from build123d import *

# Parameters (mm, degrees)
SALIENTE_EXTRUIR1_DEPTH    = 10
REDONDEO1_R                = 0.5
REDONDEO2_R                = 0.5
CROQUIS3_W                 = 6.24
CROQUIS3_H                 = 1.8
SALIENTE_EXTRUIR2_DEPTH    = 10
CROQUIS2_R                 = 1.5
CORTAR_EXTRUIR1_DEPTH      = 2.8
CORTAR_EXTRUIR1_DEPTH_BACK = 5.3


with BuildPart() as part:
    # Croquis1 → Saliente-Extruir1 (new body)
    with BuildSketch(Plane(origin=(0, 0, 0), x_dir=(-1, 0, 0), z_dir=(0, 0, 1))):
        Polygon((4.5, -1.799339828), (4.5, -3.439339828), (7.16, -6.099339828), (9.75, -6.099339828), (12.84, -6.099339828), (15.5, -3.439339828), (15.5, -1.799339828), align=None)
    extrude(amount=SALIENTE_EXTRUIR1_DEPTH)

    # Redondeo1
    redondeo1_edges = [part.edges().sort_by_distance(p)[0] for p in [
        (-15.5, 1.799339828, 5),
    ]]
    fillet(redondeo1_edges, radius=REDONDEO1_R)

    # Redondeo2
    redondeo2_edges = [part.edges().sort_by_distance(p)[0] for p in [
        (-15.5, 3.439339828, 5),
        (-12.84, 6.099339828, 5),
        (-7.16, 6.099339828, 5),
        (-4.5, 3.439339828, 5),
        (-4.5, 1.799339828, 5),
    ]]
    fillet(redondeo2_edges, radius=REDONDEO2_R)

    # Croquis3 → Saliente-Extruir2 (add)
    with BuildSketch(Plane.XY.offset(10)):
        with Locations((-10, 0.899339828)):
            Rectangle(CROQUIS3_W, CROQUIS3_H)
    extrude(amount=-SALIENTE_EXTRUIR2_DEPTH)

    # Croquis2 → Cortar-Extruir1 (cut, two sides)
    with BuildSketch(Plane(origin=(0, 1.799339828, 0), x_dir=(-1, 0, 0), z_dir=(0, -1, 0))) as cortar_extruir1_sk:
        with Locations((10, -5)):
            Circle(CROQUIS2_R)
    extrude(amount=CORTAR_EXTRUIR1_DEPTH, mode=Mode.SUBTRACT)
    extrude(cortar_extruir1_sk.sketch, amount=-CORTAR_EXTRUIR1_DEPTH_BACK, mode=Mode.SUBTRACT)


solid = part.part
Read the model definition and answer for the solid it produces. Units are mm, in the model's axes. A direction names the side the tool comes from. Give positions to 0.01 mm unless a question says otherwise; leave off trailing zeros. Write each loop counter-clockwise with the first axis right and the second up, starting at its lowest first coordinate (ties: lowest second). Pieces come first, ordered by that corner, then holes. Notation, with made-up numbers: M 61,71 L 108,71 A31 ccw 108,101 Z; hole C 49.25,-6 d3. An arc over 180 degrees is marked long. One line per item, written item: value. Start each with the question number.
(1) Find section B-B (z = 5). Determine the outline of the cut face in (x, y).
(2) A tool of negligible diameter and unlimited length cuts with its end or side. For faces 1 (the flat face through (-10, 3, 10)), 2 (the flat face through (-13.12, 1, 5)), 3 (the flat face through (-6.88, 1, 5)), from which of +Z, -Z, +X, -X, +Y, -Y can it reach the whole face along a straight path? Write none if from no direction.
(3) Find the intervals of material crossed by line 1 (Z direction, x = -10, y = 1.05); line 2 (X direction, y = 1.15, z = 5); line 3 (Z direction, x = -10.75, y = 4.25), in increasing order.
(4) Find section C-C (y = 3). Determine the outline of the cut face in (x, z), plus the area to 3 significant figures.
(5) Find section D-D (z = 9). Determine the outline of the cut face in (x, y), plus the area to 3 significant figures.
(6) Flat-ended cylindrical pins translate along their axes: pin 1 Ø0.9 at (y, z) = (0.5, 7.5) entering from -X; pin 2 Ø0.5 at (y, z) = (0.5, 6) entering from +X; pin 3 Ø0.9 at (x, z) = (-14.5, 7.5) entering from -Y; pin 4 Ø5 at (x, z) = (-10, 5) entering from +Y. Find the tip coordinate at first contact, or state that the pin passes through.
(7) Find section A-A (x = -10). Determine the outline of the cut face in (y, z).
Results below:
1. outline: M -15.5,2.3 A0.5 ccw -15,1.8 L -13.12,1.8 L -13.12,0 L -11.5,0 L -11.5,6.1 L -12.63,6.1 A0.5 ccw -12.99,5.95 L -15.35,3.59 A0.5 ccw -15.5,3.23 Z; M -8.5,0 L -6.88,0 L -6.88,1.8 L -5,1.8 A0.5 ccw -4.5,2.3 L -4.5,3.23 A0.5 ccw -4.65,3.59 L -7.01,5.95 A0.5 ccw -7.37,6.1 L -8.5,6.1 Z
2. face 1: +Z, +X, -X, +Y, -Y
2. face 2: +Z, -Z, -X, -Y
2. face 3: +Z, -Z, +X, -Y
3. line 1: z = 0 to 3.5, 6.5 to 10
3. line 2: x = -13.12 to -11.5, -8.5 to -6.88
3. line 3: z = 0 to 3.7, 6.3 to 10
4. outline: M -15.5,0 L -4.5,0 L -4.5,10 L -15.5,10 Z; hole C -10,5 d3
4. area: 103 mm^2
5. outline: M -15.5,2.3 A0.5 ccw -15,1.8 L -13.12,1.8 L -13.12,0 L -6.88,0 L -6.88,1.8 L -5,1.8 A0.5 ccw -4.5,2.3 L -4.5,3.23 A0.5 ccw -4.65,3.59 L -7.01,5.95 A0.5 ccw -7.37,6.1 L -12.63,6.1 A0.5 ccw -12.99,5.95 L -15.35,3.59 A0.5 ccw -15.5,3.23 Z
5. area: 51.3 mm^2
6. pin 1: stops at x = -13.12
6. pin 2: stops at x = -6.88
6. pin 3: stops at y = 1.8
6. pin 4: stops at y = 6.1
7. outline: M 0,0 L 6.1,0 L 6.1,3.5 L 0,3.5 Z; M 0,6.5 L 6.1,6.5 L 6.1,10 L 0,10 Z
